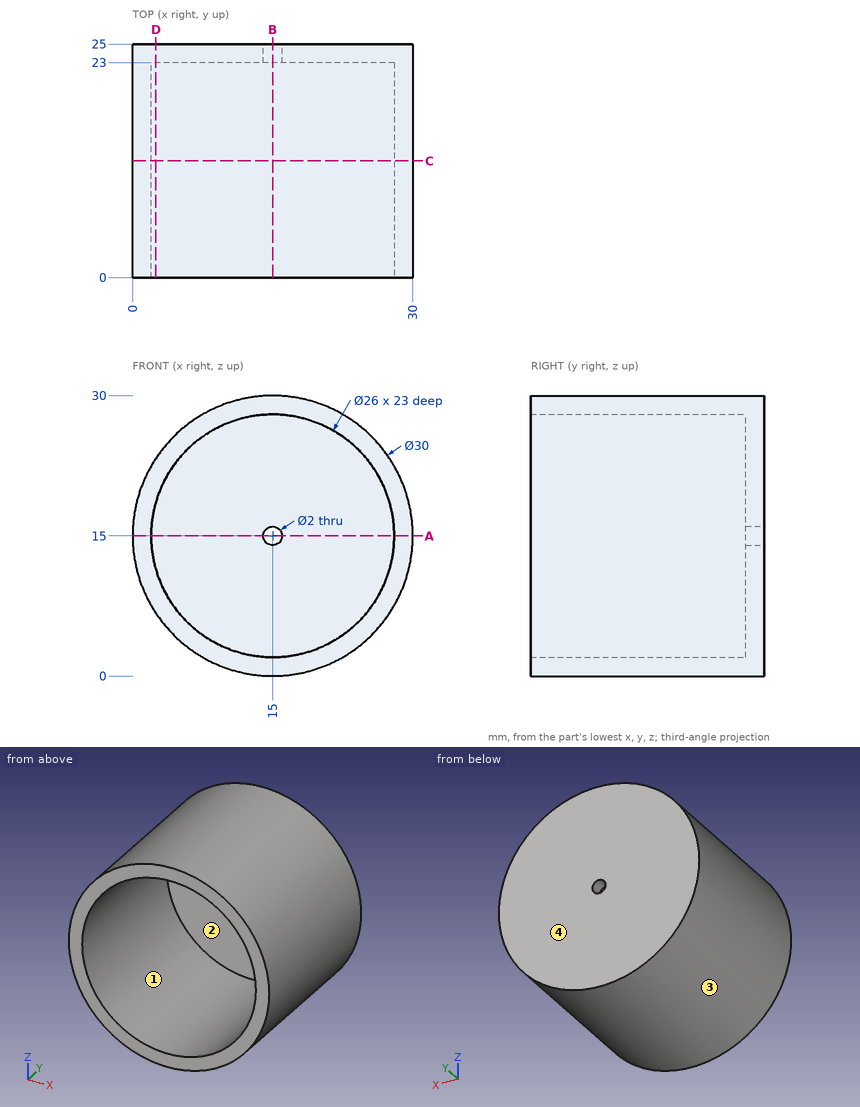
Can you work these out from the drawing? Everything is in mm from the part's minimum corner. Give positions to 0.01 mm unless a question says otherwise; leave off trailing zeros. Loops run counter-clockwise (first coordinate to the right, second up) from the corner with the lowest first, then second, coordinate; pieces in that order, holes last. Notation, with made-up numbers: M 55.25,36 L 111.25,36 A16 ccw 111.25,60 Z; hole C 54.25,-34.5 d8. An arc over 180 degrees is marked long. Put each result on its own line as item: value. Start each with the question number.
(1) I want a section at C-C on y = 12.5. Please give me the cut outline in (x, z), then the cut area to 3 significant figures.
(2) I want a section at D-D on x = 2.5. Please give me the cut outline in (y, z).
(3) I need wall thicknesses on line 1 along Z through (x, y) = (15, 13.25); line 2 along Z through (x, y) = (15, 24.55); line 3 along Y through (x, z) = (20, 10). Which ranges of each line are inside material? Lowest first, please. Write a range as [from, to].
(4) If we mould it in two halves opening along Z, with no side actions, what happens to the marked faces 1, 2, 3 and 4? For each: +Z half, -Z half, draft (parallel to the pull), parting line (faces both ways), or undercut.
(5) I want a section at B-B on x = 15. Please give me the cut outline in (y, z).
(6) I want a section at A-A on z = 15. Please give me the cut outline in (x, y).
(7) Will these pins go through, and if not, where does the flat tip stop? pin 1 Ø13 at (x, z) = (14.5, 18.5) entering from -Y; pin 2 Ø6 at (x, y) = (25, 14) entering from +Z; pin 3 Ø8 at (y, z) = (3.5, 3) entering from -X; pin 4 Ø12 at (x, z) = (6, 13.5) entering from -Y.
Answer block:
1. outline: C 15,15 d30; hole C 15,15 d26
1. area: 176 mm^2
2. outline: M 0,6.71 L 25,6.71 L 25,23.29 L 0,23.29 L 0,18.57 L 23,18.57 L 23,11.43 L 0,11.43 Z
3. line 1: [0, 2], [28, 30]
3. line 2: [0, 14], [16, 30]
3. line 3: [23, 25]
4. face 1: undercut
4. face 2: undercut
4. face 3: parting line
4. face 4: draft
5. outline: M 0,0 L 25,0 L 25,14 L 23,14 L 23,2 L 0,2 Z; M 0,28 L 23,28 L 23,16 L 25,16 L 25,30 L 0,30 Z
6. outline: M 0,0 L 2,0 L 2,23 L 14,23 L 14,25 L 0,25 Z; M 16,23 L 28,23 L 28,0 L 30,0 L 30,25 L 16,25 Z
7. pin 1: y = 23
7. pin 2: z = 28.27
7. pin 3: x = 2.31
7. pin 4: y = 0
